```python
from build123d import *
from build123d.topology import SkipClean

# Parameters (mm, degrees)
BOSS_EXTRUDE2_DEPTH = 5
CIRPATTERN1_COUNT   = 4
SKETCH5_R           = 1.5
CUT_EXTRUDE1_DEPTH  = 10
CUT_EXTRUDE2_DEPTH  = 10
SKETCH8_W           = 5.65
SKETCH8_H           = 2.5
CUT_EXTRUDE3_DEPTH  = 6.5
SKETCH10_R          = 1.5
CUT_EXTRUDE5_DEPTH  = 10
CUT_EXTRUDE6_START  = -10
CUT_EXTRUDE6_DEPTH  = 10
SKETCH13_W          = 5.7
SKETCH13_H          = 2.5
CUT_EXTRUDE7_DEPTH  = 7.5


with BuildPart() as part:
    # Sketch3 → Revolve1 (revolve)
    with BuildSketch(Plane(origin=(0, 0, 0), x_dir=(0, 0, -1), z_dir=(1, 0, 0)), mode=Mode.PRIVATE) as revolve1_sk:
        Polygon((-7.337359925, 0), (14.162640075, 0), (14.162640075, -3.75), (4.162640075, -3.75), (4.162640075, -6.25), (16.162640075, -6.25), (21.162640075, -6.25), (21.162640075, -3.047373414), (21.162640075, 4.75), (19.162640075, 4.75), (-7.337359925, 4.75), align=None)
    revolve(revolve1_sk.sketch.rotate(Axis((0, 4.75, 26.894611834), (0, 0, -1)), 270), axis=Axis((0, 4.75, 26.894611834), (0, 0, -1)))

    # Sketch4 → Boss-Extrude2 (add)
    with SkipClean():  # the faces are left unmerged after this step: merging them gives an invalid solid
        with BuildSketch(Plane.XY.offset(-4.162640075)):
            with BuildLine():
                Line((-1.948133817, 15.576115399), (-1.542950524, 13.108786017))
                ThreePointArc((-1.542950524, 13.108786017), (-3.700532064, 12.402193309), (-5.594111688, 11.149680807))
                Line((-5.594111688, 11.149680807), (-7.239438655, 13.031939867))
                ThreePointArc((-7.239438655, 13.031939867), (-4.766663326, 14.663572552), (-1.948133817, 15.576115399))
            make_face()
        boss_extrude2 = extrude(amount=BOSS_EXTRUDE2_DEPTH)

    # CirPattern1: Boss-Extrude2 ×4 about axis
    with SkipClean():  # the faces are left unmerged after this step: merging them gives an invalid solid
        cirpattern1_axis = Axis((0, 4.75, 0), (0, 0, 1))
        for i in range(1, CIRPATTERN1_COUNT):
            add(boss_extrude2.rotate(cirpattern1_axis, i * 360 / CIRPATTERN1_COUNT))

    # Sketch5 → Cut-Extrude1 (cut)
    with SkipClean():  # the faces are left unmerged after this step: merging them gives an invalid solid
        with BuildSketch(Plane.XY.offset(7.337359925)):
            with Locations((0, 4.75)):
                Circle(SKETCH5_R)
        extrude(amount=-CUT_EXTRUDE1_DEPTH, mode=Mode.SUBTRACT)

    # Sketch7 → Cut-Extrude2 (cut)
    with SkipClean():  # the faces are left unmerged after this step: merging them gives an invalid solid
        with BuildSketch(Plane(origin=(0, 0, -21.162640075), x_dir=(-1, 0, 0), z_dir=(0, 0, -1))):
            with BuildLine():
                Line((-1.445, 6.273802809), (1.445, 6.273802809))
                ThreePointArc((1.445, 6.273802809), (0, 2.65), (-1.445, 6.273802809))
            make_face()
        extrude(amount=-CUT_EXTRUDE2_DEPTH, mode=Mode.SUBTRACT)

    # Sketch8 → Cut-Extrude3 (cut)
    with SkipClean():  # the faces are left unmerged after this step: merging them gives an invalid solid
        with BuildSketch(Plane(origin=(0, 0, -21.162640075), x_dir=(-1, 0, 0), z_dir=(0, 0, -1))):
            with Locations((0, 8.523802809)):
                Rectangle(SKETCH8_W, SKETCH8_H)
        extrude(amount=-CUT_EXTRUDE3_DEPTH, mode=Mode.SUBTRACT)

    # Sketch10 → Cut-Extrude5 (cut)
    with SkipClean():  # the faces are left unmerged after this step: merging them gives an invalid solid
        with BuildSketch(Plane.XZ.offset(-6.273802809)):
            with Locations(Location((0, -18.162640075, 0), (0, 0, 270))):
                Circle(SKETCH10_R)
        extrude(amount=-CUT_EXTRUDE5_DEPTH, mode=Mode.SUBTRACT)

    # Sketch12 → Cut-Extrude6 (cut)
    with SkipClean():  # the faces are left unmerged after this step: merging them gives an invalid solid
        with BuildSketch(Plane.XY.offset(7.337359925).offset(CUT_EXTRUDE6_START)):
            with BuildLine():
                Line((-1.907535842, 9.100150229), (1.907535842, 9.100150229))
                ThreePointArc((1.907535842, 9.100150229), (0, 9.5), (-1.907535842, 9.100150229))
            make_face()
        extrude(amount=CUT_EXTRUDE6_DEPTH, mode=Mode.SUBTRACT)

    # Sketch13 → Cut-Extrude7 (cut)
    with SkipClean():  # the faces are left unmerged after this step: merging them gives an invalid solid
        with BuildSketch(Plane(origin=(0, 9.100150229, 0), x_dir=(1, 0, 0), z_dir=(0, 1, 0))):
            with Locations((0, -3.015381777)):
                Rectangle(SKETCH13_W, SKETCH13_H)
        extrude(amount=-CUT_EXTRUDE7_DEPTH, mode=Mode.SUBTRACT)


solid = part.part
```
Build history of the part. All positions in model axes, mm. A direction names the side the tool comes from. Give positions to 0.01 mm unless a question says otherwise; leave off trailing zeros. Loops run counter-clockwise (first coordinate to the right, second up) from the corner with the lowest first, then second, coordinate; pieces in that order, holes last. Notation, with made-up numbers: (14, 74) -> (67, 74) arc R26 cw to (67, 112) -> close; hole circle Ø3 at (-19, 58.25). An arc over 180 degrees is marked (long way). One line per question, with ' | ' between items.
Q1. Drop flat-ended pins along their axis: pin 1 (5 mm diameter, centred on x = 3.5, y = -3, fed in from +Z); pin 2 (4 mm diameter, centred on x = 8, z = -2, fed in from -Y); pin 3 (3 mm diameter, centred on y = 4, z = 3, fed in from +X). Give the stop position or say it passes through.
Filled sheet:
pin 1: stops at z = 0.84 | pin 2: stops at y = -4.47 | pin 3: stops at x = 4.75
Q2. Pull direction X, two halves, no side cores. Call faces 1 (the flat face through (0, 1.6, 3)), 2 (the flat face through (-1, 3, 7.337)), 3 (the flat face through (-6.405, 12.078, -1.698)): pulls with the +X half, pulls with the -X half, needs draft (parallel to the pull), parting line crosses it, or undercut.
Filled sheet:
face 1: undercut | face 2: needs draft | face 3: pulls with the -X half
Q3. Tool access for faces 4 (the flat face through (-1.75, 14.36, -1.7)), 5 (the cylindrical face through (-0.62, 0.04, -3.56)), 6 (the flat face through (0, 6.274, -14)), 7 (the cylindrical face through (0.451, 6.767, -19.593)): list every direction of +Z, -Z, +X, -X, +Y, -Y with a clear straight run to the whole face (end or side of a thin tool).
Filled sheet:
face 4: +Z, +X, +Y | face 5: +Z | face 6: -Z | face 7: +Y
Q4. Cut at A-A, the plane y = 14. Write the cut outline in (x, z), plus the area to 3 significant figures.
Filled sheet:
outline: (-5.95, -21.16) -> (5.95, -21.16) -> (5.95, -4.16) -> (-1.69, -4.16) -> (-1.69, 0.84) -> (-5.95, 0.84) -> close; hole circle Ø3 at (0, -18.16) | area: 217 mm²
Q5. Cut at D-D, the plane y = 4.75. Write the cut outline in (x, z).
Filled sheet:
outline: (-11, -21.16) -> (-2.1, -21.16) -> (-2.1, -11.16) -> (2.1, -11.16) -> (2.1, -21.16) -> (11, -21.16) -> (11, -4.16) -> (8.5, -4.16) -> (8.5, -14.16) -> (4.75, -14.16) -> (4.75, 7.34) -> (1.5, 7.34) -> (1.5, 4.27) -> (2.85, 4.27) -> (2.85, 1.77) -> (1.5, 1.77) -> (1.5, -2.66) -> (-1.5, -2.66) -> (-1.5, 1.77) -> (-2.85, 1.77) -> (-2.85, 4.27) -> (-1.5, 4.27) -> (-1.5, 7.34) -> (-4.75, 7.34) -> (-4.75, -14.16) -> (-8.5, -14.16) -> (-8.5, -4.16) -> (-11, -4.16) -> close
Q6. Cut at C-C, the plane z = -8. Write the cut outline in (x, y).
Filled sheet:
outline: circle Ø22 at (0, 4.75); circle Ø9.5 at (0, 4.75); hole circle Ø17 at (0, 4.75)
Q7. Drill centre lines: line 1 along Z through (x, y) = (0, 6.5); line 2 along Y through (x, z) = (-0.5, -6); line 3 along Y through (x, z) = (-2, -7). Where is each one in solid material? Low to high. Write a range as [from, to].
Filled sheet:
line 1: z = [-21.16, -19.66], [-16.66, 1.77], [4.27, 7.34] | line 2: y = [-6.24, -3.74], [0.03, 9.47], [13.24, 15.74] | line 3: y = [-6.07, -3.51], [0.44, 9.06], [13.01, 15.57]
Q8. Cut at B-B, the plane x = 0. Count the separate pieces of the cut face and the enclosed holes in it, plus the area to 3 significant figures.
Filled sheet:
separate pieces: 4 | enclosed holes: 0 | area: 290 mm²
